Source: CAD feature listing. Evaluate the final solid. Frame: model axes, mm. A direction names the side the tool comes from. Round coordinates to 2 decimals unless told otherwise and drop trailing zeros. Write each loop counter-clockwise with the first axis right and the second up, starting at its lowest first coordinate (ties: lowest second). Pieces come first, ordered by that corner, then holes.
```python
from build123d import *

# Parameters (mm, degrees)
F0_R     = 1.09933
F1_DEPTH = 3.175


with BuildPart() as f1:
    # F0 (on Top) → F1 (new body)
    with BuildSketch(Plane.XY):
        with BuildLine():
            Line((-28.183714, 20.612877), (-28.183714, -9.387123))
            Line((-28.183714, -9.387123), (-6.471708, -9.387123))
            Line((-6.471708, -9.387123), (-6.471708, -12.562123))
            Line((-6.471708, -12.562123), (3.528292, -12.562123))
            Line((3.528292, -12.562123), (3.528292, -9.387123))
            Line((3.528292, -9.387123), (25.240297, -9.387123))
            Line((25.240297, -9.387123), (25.240297, 20.612877))
            ThreePointArc((25.240297, 20.612877), (-1.471708, 47.324882), (-28.183714, 20.612877))
        make_face()
        with Locations((-5.796011, 2.705928)):
            Circle(F0_R, mode=Mode.SUBTRACT)
        with Locations((2.852595, 2.705928)):
            Circle(F0_R, mode=Mode.SUBTRACT)
        with BuildLine():
            ThreePointArc((-23.183714, 20.612877), (-1.471708, 42.324882), (20.240297, 20.612877))
            Line((20.240297, 20.612877), (20.240297, 9.01164))
            ThreePointArc((20.240297, 9.01164), (19.654511, 7.597426), (18.240297, 7.01164))
            Line((18.240297, 7.01164), (-21.183714, 7.01164))
            ThreePointArc((-21.183714, 7.01164), (-22.597927, 7.597426), (-23.183714, 9.01164))
            Line((-23.183714, 9.01164), (-23.183714, 20.612877))
        make_face(mode=Mode.SUBTRACT)
    extrude(amount=F1_DEPTH)


solid = f1.part
```
Q1. Section query B-B, the plane x = -22. Output: boundary loops of the cut face in (y, z) (3 decimals), and give its area (3 significant figures).
Q2. Mould query, pull axis X, two halves, no side actions, for faces 1 (the face through (-2, 4, 3.175)), 2 (the face through (-23.184, 15, 2)), 3 (the face through (-22.6, 7.6, 1.6)), 4 (the face through (3.528, -11, 2)). Classes: pulls with the +X half, pulls with the -X half, needs draft (parallel to the pull), parting line crosses it, or undercut.
Q3. Section query D-D, the plane x = 21. Output: boundary loops of the cut face in (y, z) (3 decimals).
Q4. Pin query (flat end, axial travel): P1, Ø1, axis at y = 27, z = 1.5, coming from the -X side; P2, Ø1, axis at y = -10.5, z = 2, coming from the +X side; P3, Ø1, axis at x = -22.5, z = 1, coming from the +Y side. Return the tip coordinate at first contact, or that it passes through.
Q5. Line query: line 1 (X direction, y = 20.5, z = 1.3); line 2 (Y direction, x = -2, z = 0.65); line 3 (Y direction, x = -13, z = 0.6). Output: solid intervals per line, ascending.
Q6. Section query C-C, the plane z = 2.35. Output: boundary loops of the cut face in (x, y).
Q7. Section query A-A, the plane y = 15. Output: boundary loops of the cut face in (x, z) (3 decimals), and give its area (4 significant figures).
Q8. Set-up query: faces 5 (the face through (19.67, 7.613, 1.565)), 6 (the face through (-17, -9.387, 2)), 7 (the face through (-28.184, 6, 2)), 8 (the face through (14, -9.387, 2)). Return all of +Z, -Z, +X, -X, +Y, -Y with unobstructed straight access to the full face (end or side cutting, diameter ignored); none if empty.
Filled in:
1. outline: (-9.387, 0) - (7.186, 0) - (7.186, 3.175) - (-9.387, 3.175) - close; (27.684, 0) - (37.704, 0) - (37.704, 3.175) - (27.684, 3.175) - close
1. area: 84.4 mm2
2. face 1: needs draft
2. face 2: undercut
2. face 3: undercut
2. face 4: pulls with the +X half
3. outline: (-9.387, 0) - (35.054, 0) - (35.054, 3.175) - (-9.387, 3.175) - close
4. P1: stops at x = -27.53
4. P2: stops at x = 3.53
4. P3: stops at y = 37.7
5. line 1: x = -28.18 to -23.18, 20.24 to 25.24
5. line 2: y = -12.56 to 7.01, 42.32 to 47.32
5. line 3: y = -9.39 to 7.01, 39.01 to 44.71
6. outline: (-28.18, -9.39) - (-6.47, -9.39) - (-6.47, -12.56) - (3.53, -12.56) - (3.53, -9.39) - (25.24, -9.39) - (25.24, 20.61) arc R26.71 ccw to (-28.18, 20.61) - close; hole (-23.18, 9.01) arc R2 ccw to (-21.18, 7.01) - (18.24, 7.01) arc R2 ccw to (20.24, 9.01) - (20.24, 20.61) arc R21.71 ccw to (-23.18, 20.61) - close; hole circle Ø2.2 at (-5.8, 2.71); hole circle Ø2.2 at (2.85, 2.71)
7. outline: (-28.184, 0) - (-23.184, 0) - (-23.184, 3.175) - (-28.184, 3.175) - close; (20.24, 0) - (25.24, 0) - (25.24, 3.175) - (20.24, 3.175) - close
7. area: 31.75 mm2
8. face 5: +Z, -Z
8. face 6: +Z, -Z, -X, -Y
8. face 7: +Z, -Z, -X, +Y, -Y
8. face 8: +Z, -Z, +X, -Y
